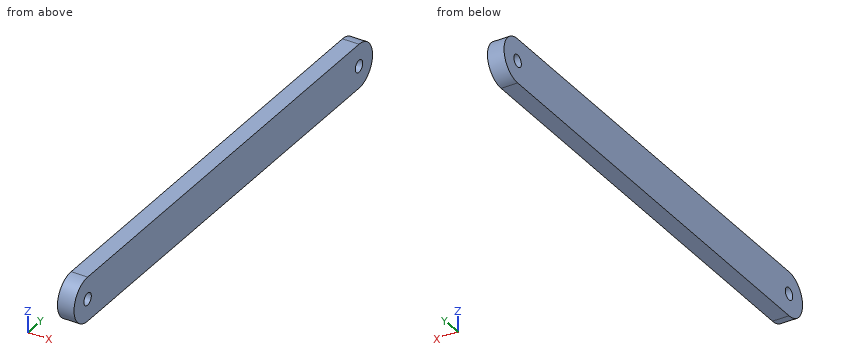
Solid Edge part; units mm, degrees
sketch "Sketch1" plane through (0, 0, 0) normal (1, 0, 0) x (0, 1, 0)
  line L0 (58.9846, 59.6775) -> (-21.0249, 59.9853)
  line L1 (-20.9941, 67.9853) -> (59.0154, 67.6774)
  arc A0 (-21.0249, 59.9853) -> (-20.9941, 67.9853) centre (-21.0095, 63.9853) cw
  arc A1 (59.0154, 67.6775) -> (58.9846, 59.6775) centre (59, 63.6775) cw
  circle A2 centre (-21.0095, 63.9853) radius 1.1
  circle A3 centre (59, 63.6775) radius 1.1
extrude "Protrusion1" add sketch "Sketch1" along normal blind 3
Here's how the part is built. I have some questions about the finished solid (model axes, mm). Coordinates: 2 decimals unless noted, no trailing zeros. Loops run counter-clockwise (first coordinate to the right, second up) from the corner with the lowest first, then second, coordinate; pieces in that order, holes last. Notation, with made-up numbers: (12.25, 71) -> (53.25, 71) arc R12 cw to (53.25, 89) -> close; hole circle Ø4 at (4, -22). An arc over 180 degrees is marked (long way). Return JSON: item names as keys, results as strings.
1) If we section it at B-B, the plane z = 61.5: Write out the boundary of the cut face in (x, y).
Results below:
{"outline": "(0, -24.14) -> (3, -24.14) -> (3, 62.36) -> (0, 62.36) -> close"}
2) If we section it at C-C, the plane y = 32: Write out the boundary of the cut face in (x, z), then the cut area to 3 significant figures.
Results below:
{"outline": "(0, 59.78) -> (3, 59.78) -> (3, 67.78) -> (0, 67.78) -> close", "area": "24.0 mm²"}
3) I need wall thicknesses on line 1 (Y direction, x = 1.9, z = 64.5); line 2 (Y direction, x = 1.6, z = 63.5); line 3 (Z direction, x = 1.25, y = 59). Which ranges of each line are inside material? Lowest first, please. Write a range as from..to.
Results below:
{"line 1": "-24.98..-21.98, -20.04..58.27, 59.73..62.91", "line 2": "-24.98..-22, -20.02..57.91, 60.09..63", "line 3": "59.68..62.58, 64.78..67.68"}
4) Will these pins go through, and if not, where does the flat tip stop? pin 1 (1.3 mm diameter, centred on y = 59, z = 63.68, fed in from +X); pin 2 (4 mm diameter, centred on y = 53, z = 63, fed in from -X); pin 3 (1 mm diameter, centred on x = 2.5, z = 67, fed in from -Y).
Results below:
{"pin 1": "through", "pin 2": "x = 0", "pin 3": "y = -24.12"}
5) If we section it at A-A, the plane x = 1.65: Write out the boundary of the cut face in (y, z), then the cut area to 3 significant figures.
Results below:
{"outline": "(-21.02, 59.99) -> (58.98, 59.68) arc R4 ccw to (59.02, 67.68) -> (-20.99, 67.99) arc R4 ccw to start; hole circle Ø2.2 at (-21.01, 63.99); hole circle Ø2.2 at (59, 63.68)", "area": "683 mm²"}
